from build123d import *

# Parameters (mm, degrees)
F0_W     = 3.175
F0_H     = 12.7
F1_DEPTH = 3.175


with BuildPart() as f1:
    # F0 (on Front) → F1 (new body)
    with BuildSketch(Plane.XZ):
        with Locations((-74.6125, 6.35)):
            Rectangle(F0_W, F0_H)
        with BuildLine():
            Line((-73.025, 0), (-38.1, 0))
            Line((-38.1, 0), (-38.1, 15.6845))
            ThreePointArc((-38.1, 15.6845), (-41.4655, 19.05), (-38.1, 22.4155))
            Line((-38.1, 22.4155), (-38.1, 38.1))
            Line((-38.1, 38.1), (-73.025, 38.1))
            Line((-73.025, 38.1), (-73.025, 25.4))
            Line((-73.025, 25.4), (-73.025, 12.7))
            Line((-73.025, 12.7), (-73.025, 0))
        make_face()
        with Locations((-74.6125, 31.75)):
            Rectangle(F0_W, F0_H)
        with BuildLine():
            Line((-38.1, 0), (-3.175, 0))
            Line((-3.175, 0), (-3.175, 12.7))
            Line((-3.175, 12.7), (-3.175, 25.4))
            Line((-3.175, 25.4), (-3.175, 38.1))
            Line((-3.175, 38.1), (-38.1, 38.1))
            Line((-38.1, 38.1), (-38.1, 22.4155))
            ThreePointArc((-38.1, 22.4155), (-35.720232, 21.429768), (-34.7345, 19.05))
            ThreePointArc((-34.7345, 19.05), (-35.720232, 16.670232), (-38.1, 15.6845))
            Line((-38.1, 15.6845), (-38.1, 0))
        make_face()
        with Locations((-1.5875, 6.35)):
            Rectangle(F0_W, F0_H)
        with Locations((-1.5875, 31.75)):
            Rectangle(F0_W, F0_H)
    extrude(amount=F1_DEPTH)


solid = f1.part
The model under review builds one solid part; all positions refer to its coordinate system, in mm. A direction names the side the tool comes from. Round coordinates to 2 decimals unless told otherwise and drop trailing zeros. One line per question, with ' | ' between items. Start each with the question number.
Item 1: Wall thickness on line 1 along Z through (x, y) = (-36.5, -1.8); line 2 along X through (y, z) = (-2.25, 15.5) (3 decimals); line 3 along X through (y, z) = (-2.15, 18.5) (3 decimals): over which ranges is each line inside the solid? List them lowest first. Write a range as [from, to].
Item 2: Draft analysis for pull direction Z (two halves, no side actions). For faces 1 (the face through (-3.175, -2, 19)), 2 (the face through (-39, -2, 0)), 3 (the face through (-76.2, -2, 6)), state which applies: +Z half, -Z half, draft (parallel to the pull), parting line (faces both ways), or undercut.
Item 3: Machinability: for faces 4 (the face through (0, -2, 32)), 5 (the face through (-75, -2, 25.4)), 6 (the face through (-2, -2, 25.4)), which of the approach directions +Z, -Z, +X, -X, +Y, -Y give a long, thin tool a straight path to every point of the face, cutting with its end or side? Answer none if there is none.
Item 4: For pin 1 (1.6 mm diameter, centred on y = -2, z = 21.5, fed in from -X) (3 decimals); pin 2 (1 mm diameter, centred on y = -2, z = 18.5, fed in from +X) (3 decimals), all flat-tipped, find the tip position at first contact; note any pin that passes through.
Return value:
1) line 1: z = [0, 16.09], [22.01, 38.1] | line 2: x = [-73.025, -3.175] | line 3: x = [-73.025, -41.42], [-34.78, -3.175]
2) face 1: undercut | face 2: -Z half | face 3: draft
3) face 4: +Z, -Z, +X, +Y, -Y | face 5: -X, +Y, -Y | face 6: +X, +Y, -Y
4) pin 1: stops at x = -73.025 | pin 2: stops at x = -3.175
